For this review, take the finished solid that the model builds, in its own axes (mm). A direction names the side the tool comes from. Coordinates: 2 decimals unless noted, no trailing zeros. Write each loop counter-clockwise with the first axis right and the second up, starting at its lowest first coordinate (ties: lowest second). Pieces come first, ordered by that corner, then holes. Notation, with made-up numbers: (-2, -38.5) - (16, -38.5) arc R18 ccw to (16, -25.5) - close; hole circle Ø2 at (-35.5, 52.25). An arc over 180 degrees is marked (long way). Use one line per item in the form item = value. Start each with the question number.
1) For L1, parallel to Z at x = -20, y = -13; L2, parallel to X at y = 3, z = 9; L3, parallel to X at y = -10, z = 7.25, list the stretches that pass through material, from the lowest coordinate up. Write a range as from..to.
2) Mouldability with a two-part tool opening along X and no side actions: class faces 4 (the flat face through (14.59, 13, 11)), 5 (the flat face through (0, 0, 0)), 6 (the cylindrical face through (-14.539, -1.528, 11.519)), 7 (the cylindrical face through (23.95, -14.35, 2.58)) as pulls with the +X half, pulls with the -X half, needs draft (parallel to the pull), parting line crosses it, or undercut.
3) We need section A-A (y = 4.5). Give the boundary of the cut face in (x, z), plus the area to 3 significant figures.
4) Insertion check: P1, Ø10, axis at x = -2, z = 8.5, coming from the -Y side; P2, Ø10, axis at y = 11.5, z = 14, coming from the -X side; P3, Ø6.5, axis at y = 7, z = 12, coming from the +X side; P4, Ø3, axis at x = -7, y = -9.5, coming from the +Z side. Each pin has a flat end and moves straight along its axis. Give the tip position at first contact, or say it passes through.
5) We need section C-C (x = 0). Give the boundary of the cut face in (y, z) (3 decimals).
6) Tool access review of faces 1 (the flat face through (0, 13, 5.08)), 2 (the flat face through (-13.091, -10, 11)), 3 (the flat face through (19.05, 8, 11)): name each direction out of +Z, -Z, +X, -X, +Y, -Y from which nothing blocks a thin tool from reaching the whole face with its end or side.
7) We need section D-D (y = 11). Give the boundary of the cut face in (x, z), plus the area to 3 significant figures.
```python
from build123d import *

# Parameters (mm, degrees)
F0_W     = 50.8
F0_H     = 31.75
F1_DEPTH = 5.08
F3_DEPTH = 12.7
F5_DEPTH = 17.78
F6_R     = 5.08
F7_R     = 5.08
F8_SIZE  = 1.27


with BuildPart() as f1:
    # F0 (on Top) → F1 (new body)
    with BuildSketch(Plane.XY):
        Rectangle(F0_W, F0_H)
    extrude(amount=F1_DEPTH)

    # F2 (on face) → F3 (join)
    with BuildSketch(Plane.XY.offset(5.08)):
        Polygon((-14.5904901437, 15.875), (-19.05, 15.875), (-19.05, 0), (-13.0905322731, 0), (-13.0905322731, -15.875), (13.0905322731, -15.875), (13.0905322731, 0), (19.05, 0), (19.05, 15.875), (14.5904901437, 15.875), (14.5904901437, 10.2269826457), (-14.5904901437, 10.2269826457), align=None)
    extrude(amount=F3_DEPTH)

    # F4 (on face) → F5 (cut, through all)
    with BuildSketch(Plane.XY.offset(17.78)):
        with BuildLine():
            Line((-11.43, -15.875), (11.43, -15.875))
            ThreePointArc((11.43, -15.875), (0, -4.445), (-11.43, -15.875))
        make_face()
    extrude(amount=-F5_DEPTH, mode=Mode.SUBTRACT)

    # F6
    f6_edges = [f1.edges().sort_by_distance(p)[0] for p in [
        (-13.090532, 0, 11.43),
        (13.090532, 0, 11.43),
    ]]
    fillet(f6_edges, radius=F6_R)

    # F7
    f7_edges = [f1.edges().sort_by_distance(p)[0] for p in [
        (25.4, -15.875, 2.54),
        (-25.4, -15.875, 2.54),
    ]]
    fillet(f7_edges, radius=F7_R)

    # F8
    f8_edges = [f1.edges().sort_by_distance(p)[0] for p in [
        (0, -4.445, 17.78),
        (0, 10.226983, 17.78),
        (-14.59049, 13.050991, 17.78),
        (14.59049, 13.050991, 17.78),
    ]]
    chamfer(f8_edges, length=F8_SIZE)


solid = f1.part
```
Determined:
q1.L1 = 0..5.08
q1.L2 = -19.05..19.05
q1.L3 = -13.09..-9.8, 9.8..13.09
q2.face_4 = undercut
q2.face_5 = needs draft
q2.face_6 = pulls with the -X half
q2.face_7 = pulls with the +X half
q3.outline = (-25.4, 0) - (25.4, 0) - (25.4, 5.08) - (19.05, 5.08) - (19.05, 17.78) - (-19.05, 17.78) - (-19.05, 5.08) - (-25.4, 5.08) - close
q3.area = 742 mm²
q4.P1 = -6.84
q4.P2 = -19.05
q4.P3 = 19.05
q4.P4 = through
q5.outline = (-4.445, 0) - (15.875, 0) - (15.875, 5.08) - (10.227, 5.08) - (10.227, 16.51) - (8.957, 17.78) - (-3.175, 17.78) - (-4.445, 16.51) - close
q6.face_1 = +Z, +Y
q6.face_2 = +Z, -X, -Y
q6.face_3 = +Z, +X, +Y, -Y
q7.outline = (-25.4, 0) - (25.4, 0) - (25.4, 5.08) - (19.05, 5.08) - (19.05, 17.78) - (15.86, 17.78) - (14.59, 16.51) - (14.59, 5.08) - (-14.59, 5.08) - (-14.59, 16.51) - (-15.86, 17.78) - (-19.05, 17.78) - (-19.05, 5.08) - (-25.4, 5.08) - close
q7.area = 370 mm²
